Autodesk Inventor part; units mm, degrees
ref_plane "YZ Plane" through (0, 0, 0) normal (1, 0, 0) x (0, 1, 0)
ref_plane "XZ Plane" through (0, 0, 0) normal (0, 1, 0) x (-1, 0, 0)
ref_plane "XY Plane" through (0, 0, 0) normal (0, 0, 1) x (1, 0, 0)
sketch "Sketch1" plane through (0, 0, 0) normal (0, 1, 0) x (-1, 0, 0)
  line L0 (0, 0) -> (-17, 0)
  line L1 (-17, 0) -> (-17, -2)
  line L2 (-17, -2) -> (0, -2)
  line L3 (0, -2) -> (0, 0)
  line L4 (0, -18) -> (-17, -18)
  line L5 (-17, -18) -> (-17, -20)
  line L6 (-17, -20) -> (0, -20)
  line L7 (0, -20) -> (0, -18)
  line L8 (-4, -2) -> (-13, -2)
  line L9 (-13, -2) -> (-13, -18)
  line L10 (-13, -18) -> (-4, -18)
  line L11 (-4, -18) -> (-4, -2)
  dimension "d0" = 17
  dimension "d1" = 2
  dimension "d2" = 17
  dimension "d3" = 2
  dimension "d4" = 16
  dimension "d7" = 4
  dimension "d8" = 4
extrude "Extrusion1" add sketch "Sketch1" along normal blind 14 contours L3 L2 L1 L0 | L4 L7 L6 L5
extrude "Extrusion2" add sketch "Sketch1" along normal blind 2 contours L11 L4 L9 L2
properties part number "drzakCudliku"
Here's how the part is built. I have some questions about the finished solid (model axes, mm). A direction names the side the tool comes from. Round coordinates to 2 decimals unless told otherwise and drop trailing zeros. Order: outer loops, then holes, each group sorted by start corner. A loop starts at its lowest first (then second) coordinate and runs counter-clockwise, first axis right, second up. Notation, with made-up numbers: M -15,-18.75 L 24,-18.75 A9 ccw 24,-10.75 Z; hole C 48.25,6.5 d2. An arc over 180 degrees is marked long. Answer in a Markdown table with one row per item.
Item 1: Imagine slicing it at A-A, the plane y = 7.5. Write out the boundary of the cut face in (x, z), and give its area (3 significant figures).
A:
| item | result |
|---|---|
| outline | M 0,-20 L 17,-20 L 17,-18 L 0,-18 Z; M 0,-2 L 17,-2 L 17,0 L 0,0 Z |
| area | 68.0 mm2 |
Item 2: For faces 5 (the face through (13, 1, -10)), 6 (the face through (17, 7, -1)), which set-ups out of +Z, -Z, +X, -X, +Y, -Y let a thin tool reach every point of the face, with its end or its side?
A:
| item | result |
|---|---|
| face 5 | +X, +Y, -Y |
| face 6 | +Z, -Z, +X, +Y, -Y |
Item 3: If I drill on L1, parallel to Z at x = 1.5, y = 10.25; L2, parallel to Y at x = 6.25, z = -13, over which ranges is the centre line in solid material (lowest first)? Write a range as from..to.
A:
| item | result |
|---|---|
| L1 | z = -20..-18, -2..0 |
| L2 | y = 0..2 |
Item 4: Thinking about a two-plate mould opening in Z: for faces 1 (the face through (9, 14, -1)), 2 (the face through (8, 7, 0)), 3 (the face through (4, 1, -10)), 4 (the face through (9, 2, -10)), which applies, +Z half, -Z half, draft (parallel to the pull), parting line (faces both ways), or undercut?
A:
| item | result |
|---|---|
| face 1 | draft |
| face 2 | +Z half |
| face 3 | undercut |
| face 4 | undercut |
Item 5: Imagine slicing it at C-C, the plane z = -4. Write out the boundary of the cut face in (x, y).
A:
| item | result |
|---|---|
| outline | M 4,0 L 13,0 L 13,2 L 4,2 Z |
Item 6: Imagine slicing it at B-B, the plane x = 14.5. Write out the boundary of the cut face in (y, z), and give its area (3 significant figures).
A:
| item | result |
|---|---|
| outline | M 0,-20 L 14,-20 L 14,-18 L 0,-18 Z; M 0,-2 L 14,-2 L 14,0 L 0,0 Z |
| area | 56.0 mm2 |
Item 7: Imagine slicing it at D-D, the plane x = 8.25. Write out the boundary of the cut face in (y, z).
A:
| item | result |
|---|---|
| outline | M 0,-20 L 14,-20 L 14,-18 L 2,-18 L 2,-2 L 14,-2 L 14,0 L 0,0 Z |
Item 8: I'm going to push flat-ended pins straight in: pin 1 (5 mm diameter, centred on y = 8.5, z = -18, fed in from -X); pin 2 (2 mm diameter, centred on y = 0.5, z = -11, fed in from -X); pin 3 (2.5 mm diameter, centred on x = 10, z = -10, fed in from +Y); pin 4 (4 mm diameter, centred on y = 11, z = -5.5, fed in from +X). Where does each tip first touch, or does it pass through?
A:
| item | result |
|---|---|
| pin 1 | stops at x = 0 |
| pin 2 | stops at x = 4 |
| pin 3 | stops at y = 2 |
| pin 4 | passes through |
